For this review, take the finished solid that the model builds, in its own axes (mm). Face numbers are marked on the shaded views. Round coordinates to 2 decimals unless told otherwise and drop trailing zeros. Write each loop counter-clockwise with the first axis right and the second up, starting at its lowest first coordinate (ties: lowest second). Pieces come first, ordered by that corner, then holes. Notation, with made-up numbers: (87.5, 7) - (126.5, 7) arc R35 cw to (126.5, 44) - close; hole circle Ø4 at (56, 83.5). An arc over 180 degrees is marked (long way). Answer in a Markdown table with one row per item. Add a question column.
from build123d import *

# Parameters (mm, degrees)
SKETCH1_W                       = 112
SKETCH1_H                       = 35.5
BOSS_EXTRUDE1_DEPTH             = 1.2
SKETCH2_W                       = 6
SKETCH2_H                       = 6
BOSS_EXTRUDE2_DEPTH             = 2
SKETCH3_R                       = 1.1
CUT_EXTRUDE1_DEPTH              = 59.83283522
SKETCH7_W                       = 0.4
SKETCH7_H                       = 35.5
CUT_EXTRUDE5_DEPTH              = 59.83283522
AUFSATZ_LINEAR_AUSTRAGEN2_DEPTH = 2
VERRUNDUNG1_R                   = 2
SKETCH8_W                       = 5.6
SKETCH8_H                       = 35.5
CUT_EXTRUDE7_DEPTH              = 2
CHAMFER1_SIZE                   = 1.3


with BuildPart() as part:
    # Sketch1 → Boss-Extrude1 (new body)
    with BuildSketch(Plane.XY):
        Rectangle(SKETCH1_W, SKETCH1_H)
    extrude(amount=BOSS_EXTRUDE1_DEPTH)

    # Sketch2 → Boss-Extrude2 (add)
    with BuildSketch(Plane.XY.offset(1.2)):
        with Locations((-53, 14.75)):
            Rectangle(SKETCH2_W, SKETCH2_H)
        with Locations((-53, -14.75)):
            Rectangle(SKETCH2_W, SKETCH2_H)
        with Locations((53, -14.75)):
            Rectangle(SKETCH2_W, SKETCH2_H)
        with Locations((53, 14.75)):
            Rectangle(SKETCH2_W, SKETCH2_H)
    extrude(amount=BOSS_EXTRUDE2_DEPTH)

    # Sketch3 → Cut-Extrude1 (cut, through all)
    with BuildSketch(Plane.XY.offset(3.2)):
        with Locations((-53, 14.75)):
            Circle(SKETCH3_R)
        with Locations((-53, -14.75)):
            Circle(SKETCH3_R)
        with Locations((53, -14.75)):
            Circle(SKETCH3_R)
        with Locations((53, 14.75)):
            Circle(SKETCH3_R)
    extrude(amount=-CUT_EXTRUDE1_DEPTH, mode=Mode.SUBTRACT)

    # Sketch7 → Cut-Extrude5 (cut, through all)
    with BuildSketch(Plane(origin=(0, 0, 0), x_dir=(-1, 0, 0), z_dir=(0, 0, -1))):
        with Locations((-55.8, 0)):
            Rectangle(SKETCH7_W, SKETCH7_H)
        with Locations((55.8, 0)):
            Rectangle(SKETCH7_W, SKETCH7_H)
    extrude(amount=-CUT_EXTRUDE5_DEPTH, mode=Mode.SUBTRACT)

    # Skizze5 → Aufsatz-Linear austragen2 (add)
    with BuildSketch(Plane.XY.offset(1.2)):
        Polygon((-50, 11.75), (0, 0), (50, 11.75), (55.6, 11.75), (55.6, 9.984275645), (6.55686033, -1.540862177), (50, -11.75), (50, -14.831724355), (0, -3.081724355), (-50, -14.831724355), (-50, -11.75), (-6.55686033, -1.540862177), (-55.6, 9.984275645), (-55.6, 11.75), align=None)
    extrude(amount=AUFSATZ_LINEAR_AUSTRAGEN2_DEPTH)

    # Verrundung1
    verrundung1_edges = [part.edges().sort_by_distance(p)[0] for p in [
        (-6.55686033, -1.540862177, 2.2),
        (0, -3.081724355, 2.2),
        (6.55686033, -1.540862177, 2.2),
        (0, 0, 2.2),
    ]]
    fillet(verrundung1_edges, radius=VERRUNDUNG1_R)

    # Sketch8 → Cut-Extrude7 (cut)
    with BuildSketch(Plane.XY.offset(1.2)):
        with Locations((-52.8, 0)):
            Rectangle(SKETCH8_W, SKETCH8_H)
        with Locations((52.8, 0)):
            Rectangle(SKETCH8_W, SKETCH8_H)
    extrude(amount=CUT_EXTRUDE7_DEPTH, mode=Mode.SUBTRACT)

    # Chamfer1
    # the kernel refuses this chamfer: 1.3 mm, written as the material it takes off along each edge
    with BuildSketch(Plane(origin=(53, 14.75, 0), x_dir=(1, 0, 0), z_dir=(0, -1, 0))) as chamfer1_piece_1:
        Polygon((1.1, CHAMFER1_SIZE), (1.1 + CHAMFER1_SIZE, 0), (1.1, 0), align=None)
    revolve(axis=Axis((53, 14.75, 0), (0, 0, 1)), mode=Mode.SUBTRACT)
    with BuildSketch(Plane(origin=(-53, -14.75, 0), x_dir=(1, 0, 0), z_dir=(0, -1, 0))) as chamfer1_piece_2:
        Polygon((1.1 + CHAMFER1_SIZE, 0), (1.1, CHAMFER1_SIZE), (1.1, 0), align=None)
    revolve(axis=Axis((-53, -14.75, 0), (0, 0, 1)), mode=Mode.SUBTRACT)
    with BuildSketch(Plane(origin=(-53, 14.75, 0), x_dir=(1, 0, 0), z_dir=(0, -1, 0))) as chamfer1_piece_3:
        Polygon((1.1 + CHAMFER1_SIZE, 0), (1.1, CHAMFER1_SIZE), (1.1, 0), align=None)
    revolve(axis=Axis((-53, 14.75, 0), (0, 0, 1)), mode=Mode.SUBTRACT)
    with BuildSketch(Plane(origin=(53, -14.75, 0), x_dir=(1, 0, 0), z_dir=(0, -1, 0))) as chamfer1_piece_4:
        Polygon((1.1 + CHAMFER1_SIZE, 0), (1.1, CHAMFER1_SIZE), (1.1, 0), align=None)
    revolve(axis=Axis((53, -14.75, 0), (0, 0, 1)), mode=Mode.SUBTRACT)


solid = part.part
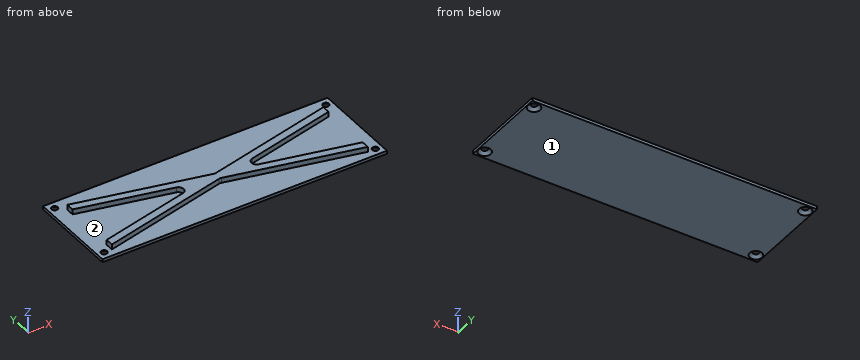
Q1. Insertion check: pin 1 Ø6 at (x, y) = (44, 5.5) entering from +Z; pin 2 Ø0.6 at (y, z) = (9.5, 2) entering from -X; pin 3 Ø1 at (x, y) = (-3, -9.5) entering from +Z. Each pin has a flat end and moves straight along its axis. Give the tip position at first contact, or say it passes through.
Q2. Add section B-B on x = -53. State the section outline as (y, z) points, then the cut area to 3 significant figures.
Q3. Add section D-D on x = 9.5. State the section outline as (y, z) points.
Q4. To check wall thickness, follow probe 1 along X at (y, z) = (-14, 1.05); probe 2 along X at (y, z) = (-14.5, 1.1); probe 3 along Z at (x, y) = (0.5, -4). State the ranges of each line that lie inside material, in increasing order.
Q5. Add section A-A on y = 14.75. State the section outline as (x, z) points.
Q6. Add section C-C on z = 2.6. State the section outline as (x, y) points, then the cut area to 3 significant figures.
Q7. Draft analysis for pull direction Y (two halves, no side actions). For the marked faces 1 and 2, state which applies: released by +Y, released by -Y, zero draft, split by the parting line, or undercut.
Answer sheet:
| question | item | result |
|---|---|---|
| 1 | pin 1 | stops at z = 3.2 |
| 1 | pin 2 | stops at x = -50 |
| 1 | pin 3 | stops at z = 1.2 |
| 2 | outline | (-17.75, 0) - (-17.15, 0) - (-15.95, 1.2) - (-17.75, 1.2) - close; (-13.55, 1.2) - (-12.35, 0) - (12.35, 0) - (13.55, 1.2) - close; (15.95, 1.2) - (17.15, 0) - (17.75, 0) - (17.75, 1.2) - close |
| 2 | area | 34.0 mm² |
| 3 | outline | (-17.75, 0) - (17.75, 0) - (17.75, 1.2) - (2.23, 1.2) - (2.23, 3.2) - (-5.31, 3.2) - (-5.31, 1.2) - (-17.75, 1.2) - close |
| 4 | probe 1 | x = -55.6 to -54.12, -51.88 to 51.88, 54.12 to 55.6 |
| 4 | probe 2 | x = -55.6 to -54.28, -51.72 to 51.72, 54.28 to 55.6 |
| 4 | probe 3 | z = 0 to 1.2 |
| 5 | outline | (-55.6, 0) - (-55.4, 0) - (-54.2, 1.2) - (-55.6, 1.2) - close; (-51.8, 1.2) - (-50.6, 0) - (50.6, 0) - (51.8, 1.2) - close; (54.2, 1.2) - (55.4, 0) - (55.6, 0) - (55.6, 1.2) - close |
| 6 | outline | (-50, -14.83) - (-0.46, -3.19) arc R2 cw to (0.46, -3.19) - (50, -14.83) - (50, -11.75) - (14.84, -3.49) arc R2 cw to (14.84, 0.41) - (50, 8.67) - (50, 11.75) - (0.46, 0.11) arc R2 cw to (-0.46, 0.11) - (-50, 11.75) - (-50, 8.67) - (-14.84, 0.41) arc R2 cw to (-14.84, -3.49) - (-50, -11.75) - close |
| 6 | area | 619 mm² |
| 7 | face 1 | zero draft |
| 7 | face 2 | undercut |
